```python
from build123d import *

# Parameters (mm, degrees)
BOSS_EXTRUDE1_DEPTH   = 64
SKETCH2_W             = 40
SKETCH2_H             = 20
CUT_EXTRUDE1_DEPTH    = 30
SKETCH3_W             = 64
SKETCH3_H             = 4.5
BOSS_EXTRUDE2_DEPTH   = 8
SKETCH4_W             = 64
SKETCH4_H             = 4.5
BOSS_EXTRUDE3_DEPTH   = 8
SKETCH5_R             = 2
CUT_EXTRUDE6_DEPTH    = 7
SKETCH6_W             = 5
SKETCH6_H             = 4.5
CUT_EXTRUDE7_DEPTH    = 7
BODY_MOVE_COPY1_ANGLE = 90
BODY_MOVE_COPY2_ANGLE = 12.4160704


with BuildPart() as part:
    # Sketch1 → Boss-Extrude1 (new body)
    with BuildSketch(Plane.XY):
        Polygon((-70.899702081, 53.100294195), (-109.964182504, 44.499923896), (-108.996640846, 40.105169848), (-69.932160423, 48.705540147), align=None)
    extrude(amount=BOSS_EXTRUDE1_DEPTH)

    # Sketch2 → Cut-Extrude1 (cut)
    with BuildSketch(Plane(origin=(-14.427653835, 65.533085344, 0), x_dir=(0.9766120105757768, 0.21500925747311134, 0), z_dir=(-0.21500925747311134, 0.9766120105757768, 0))):
        with Locations((-77.824445772, -32)):
            Rectangle(SKETCH2_W, SKETCH2_H)
    extrude(amount=-CUT_EXTRUDE1_DEPTH, mode=Mode.SUBTRACT)


with BuildPart() as cut_extrude1_piece_1:
    # of the separate pieces the step leaves, piece 1, a body of its own (cut_extrude1_pieces)
    add(part.part.solids().sort_by_distance((-70.899702081, 53.100294195, 0))[0])



with BuildPart() as cut_extrude1_piece_2:
    # of the separate pieces the step leaves, piece 2, a body of its own (cut_extrude1_pieces)
    add(part.part.solids().sort_by_distance((-70.899702081, 53.100294195, 42))[0])


with BuildPart() as cut_extrude1_piece_1_1:
    add(cut_extrude1_piece_1.part)

    add(cut_extrude1_piece_2.part)  # Boss-Extrude2 merges Cut-Extrude1 piece 2
    # Sketch3 → Boss-Extrude2 (add)
    with BuildSketch(Plane(origin=(-56.472048246, -12.432791149, 0), x_dir=(0, 0, -1), z_dir=(0.976612010575777, 0.2150092574731111, 0))):
        with Locations((-32, 64.852477375)):
            Rectangle(SKETCH3_W, SKETCH3_H)
    extrude(amount=BOSS_EXTRUDE2_DEPTH)

    # Sketch4 → Boss-Extrude3 (add)
    with BuildSketch(Plane(origin=(-95.536528669, -21.033161448, 0), x_dir=(0, 0, 1), z_dir=(-0.9766120105757774, -0.21500925747310878, 0))):
        with Locations((32, 64.852477375)):
            Rectangle(SKETCH4_W, SKETCH4_H)
    extrude(amount=BOSS_EXTRUDE3_DEPTH)

    # Sketch5 → Cut-Extrude6 (cut)
    with BuildSketch(Plane(origin=(-13.460112176, 61.138331296, 0), x_dir=(0.976612010575777, 0.21500925747311095, 0), z_dir=(0.21500925747311095, -0.976612010575777, 0))):
        with Locations((-52.824445772, 26)):
            Circle(SKETCH5_R)
        with Locations((-52.824445772, 38)):
            Circle(SKETCH5_R)
        with Locations((-102.824445772, 26)):
            Circle(SKETCH5_R)
        with Locations((-102.824445772, 38)):
            Circle(SKETCH5_R)
    extrude(amount=-CUT_EXTRUDE6_DEPTH, mode=Mode.SUBTRACT)

    # Sketch6 → Cut-Extrude7 (cut)
    with BuildSketch(Plane(origin=(-13.460112176, 61.138331296, 0), x_dir=(0.976612010575777, 0.21500925747311095, 0), z_dir=(0.21500925747311095, -0.976612010575777, 0))):
        with Locations((-57.324445772, 2.25)):
            Rectangle(SKETCH6_W, SKETCH6_H)
        with Locations((-67.324445772, 2.25)):
            Rectangle(SKETCH6_W, SKETCH6_H)
        with Locations((-77.324445772, 2.25)):
            Rectangle(SKETCH6_W, SKETCH6_H)
        with Locations((-87.324445772, 2.25)):
            Rectangle(SKETCH6_W, SKETCH6_H)
        with Locations((-97.324445772, 2.25)):
            Rectangle(SKETCH6_W, SKETCH6_H)
        with Locations((-97.324445772, 61.75)):
            Rectangle(SKETCH6_W, SKETCH6_H)
        with Locations((-87.324445772, 61.75)):
            Rectangle(SKETCH6_W, SKETCH6_H)
        with Locations((-77.324445772, 61.75)):
            Rectangle(SKETCH6_W, SKETCH6_H)
        with Locations((-67.324445772, 61.75)):
            Rectangle(SKETCH6_W, SKETCH6_H)
        with Locations((-57.324445772, 61.75)):
            Rectangle(SKETCH6_W, SKETCH6_H)
    extrude(amount=-CUT_EXTRUDE7_DEPTH, mode=Mode.SUBTRACT)


with BuildPart() as cut_extrude1_piece_1_2:
    # Body-Move/Copy1: read off the stored shape, not the designer's step
    # Body-Move/Copy1: moved
    add(cut_extrude1_piece_1_1.part.moved(Location((0, -54.8203683, 54.8203683))).rotate(Axis((0, 0, 0), (-1, 0, 0)), BODY_MOVE_COPY1_ANGLE))


with BuildPart() as cut_extrude1_piece_1_3:
    # Body-Move/Copy2: read off the stored shape, not the designer's step
    # Body-Move/Copy2: moved
    add(cut_extrude1_piece_1_2.part.moved(Location((2.9503173, 0, 14.8930484))).rotate(Axis((0, 0, 0), (0, -1, 0)), BODY_MOVE_COPY2_ANGLE))


solid = cut_extrude1_piece_1_3.part
```
Geometry: final body of the model. Coordinates: model frame, mm. A direction names the side the tool comes from. Round coordinates to 2 decimals unless told otherwise and drop trailing zeros. Order: outer loops, then holes, each group sorted by start corner. A loop starts at its lowest first (then second) coordinate and runs counter-clockwise, first axis right, second up. Notation, with made-up numbers: (13.25, 4.25) - (20.25, 4.25) arc R23 ccw to (20.25, 29.25) - close; hole circle Ø5 at (-3.5, -32). An arc over 180 degrees is marked (long way). Write item = value, one per line. Start each with the question number.
Q1. Cut plane B-B on x = -65.5. Return the cut outline in (y, z), and give its area (3 significant figures).
Q2. Access query for faces 1 (the flat face through (-106.932, 57, 4)), 2 (the flat face through (-115, 54.82, 4)), 3 (the flat face through (-89, 114.32, 4)). Directions: +Z, -Z, +X, -X, +Y, -Y. A direction counts if a zero-diameter tool reaches every point of the face in a straight line with its end or side. Return the directions, or none.
Q3. Cut plane D-D on z = 5.35. Give the number of separate pieces and of enclosed holes in the cut face, and give its area (3 significant figures).
Q4. Cut plane C-C on x = -79. Return the cut outline in (y, z), and give its area (4 significant figures).
Q5. Ray query, line 1 (X direction, y = 115.5, z = 3.15); line 2 (Y direction, x = -115, z = 4.25); line 3 (Y direction, x = -99, z = 3.55). Return the intervals inside material, ascending. Write a range as from..to.
Q6. Pull-direction query (Y, two-part tool) for faces 4 (the flat face through (-90, 76.82, 4)), 5 (the cylindrical face through (-65.37, 78.87, 3.9)), 6 (the flat face through (-74, 118.82, 4)), 7 (the flat face through (-101.932, 117, 4)); classes: +Y half, -Y half, draft (parallel to the pull), parting line (faces both ways), or undercut.
Q7. Pin query (flat end, axial travel): pin 1 (1.4 mm diameter, centred on x = -88.5, z = 4.5, fed in from -Y); pin 2 (1 mm diameter, centred on x = -81.5, z = 2, fed in from -Y); pin 3 (1.4 mm diameter, centred on x = -89.5, z = 4, fed in from +Y). Return the tip coordinate at first contact, or that it passes through.
Q8. Cut plane A-A on x = -86. Return the cut outline in (y, z), and give its area (3 significant figures).
Outcome:
q1.outline = (54.82, 1.61) - (78.9, 1.61) - (78.9, 6.11) - (54.82, 6.11) - close; (82.74, 1.61) - (90.9, 1.61) - (90.9, 6.11) - (82.74, 6.11) - close; (94.74, 1.61) - (118.82, 1.61) - (118.82, 6.11) - (94.74, 6.11) - close
q1.area = 253 mm^2
q2.face_1 = +Z, -Z, -Y
q2.face_2 = +Z, -Z, +X, -X, -Y
q2.face_3 = +Z, -Z, +Y
q3.separate_pieces = 1
q3.enclosed_holes = 5
q3.area = 2,510 mm^2
q4.outline = (59.32, 1.61) - (76.82, 1.61) - (76.82, 6.11) - (59.32, 6.11) - close; (96.82, 1.61) - (114.32, 1.61) - (114.32, 6.11) - (96.82, 6.11) - close
q4.area = 157.5 mm^2
q5.line_1 = -117.93..-111.93, -106.93..-101.93, -96.93..-91.93, -86.93..-81.93, -76.93..-71.93, -66.93..-61.93
q5.line_2 = 54.82..78.82, 82.82..90.82, 94.82..118.82
q5.line_3 = 59.32..76.82, 96.82..114.32
q6.face_4 = undercut
q6.face_5 = undercut
q6.face_6 = +Y half
q6.face_7 = draft
q7.pin_1 = 59.32
q7.pin_2 = 54.82
q7.pin_3 = 114.32
q8.outline = (54.82, 1.61) - (76.82, 1.61) - (76.82, 6.11) - (54.82, 6.11) - close; (96.82, 1.61) - (118.82, 1.61) - (118.82, 6.11) - (96.82, 6.11) - close
q8.area = 198 mm^2
